Read the model definition and answer for the solid it produces. Units are mm, in the model's axes. Face numbers are marked on the shaded views. A direction names the side the tool comes from. Coordinates: 2 decimals unless noted, no trailing zeros. Write each loop counter-clockwise with the first axis right and the second up, starting at its lowest first coordinate (ties: lowest second). Pieces come first, ordered by that corner, then holes. Notation, with made-up numbers: (21, 57) -> (63, 57) arc R19 cw to (63, 89) -> close; hole circle Ø6 at (-6.75, 76). An arc over 180 degrees is marked (long way). One line per item, written item: value. Start each with the question number.
1. Consider line 1 along Y through (x, z) = (0, 9.5); line 2 along Y through (x, z) = (-2.25, 8). Determine where each line is inside the solid, lowest interval first.
2. For a pull along Y with two mould halves and no side action, classify the marked faces 1, 2 and 3 as pulls with the +Y half, pulls with the -Y half, needs draft (parallel to the pull), parting line crosses it, or undercut.
3. Find section D-D, the plane x = -2. Write down the section's boundary in (y, z).
4. Given P1, Ø5, axis at y = 6, z = 11, coming from the -X side; P2, Ø6.5, axis at x = 0, y = 0, coming from the -Z side; P3, Ø10, axis at y = -9.5, z = 9, coming from the +X side; P4, Ø10, axis at x = -10, y = -1.5, coming from the +Z side, each flat-ended and moving along its own axis, determine where each tip first touches the part or whether it passes through.
5. For the marked faces 4 and 5, determine the directions among +Z, -Z, +X, -X, +Y, -Y from which every point of the face is accessible in a straight line to the end or side of a thin tool.
6. Find section C-C, the plane x = -11. Write down the section's boundary in (y, z).
7. Find section B-B, the plane z = 20.75. Write down the section's boundary in (x, y), and give its area (3 significant figures).
8. Find section A-A, the plane y = 10.5. Write down the section's boundary in (x, z), and give its area (3 significant figures).
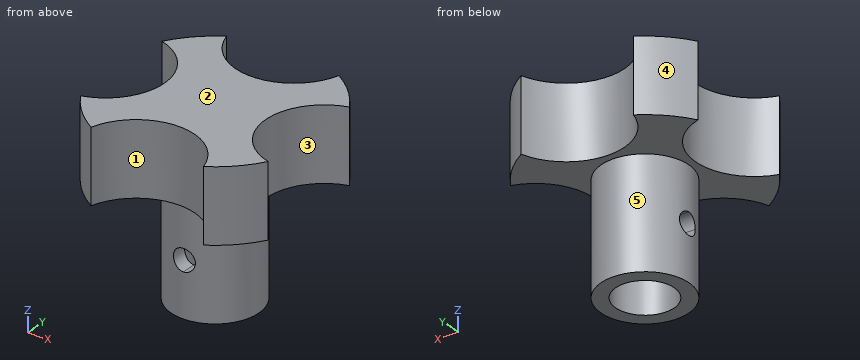
```python
from build123d import *

# Parameters (mm, degrees)
IZIM1_R                     = 6
IZIM1_R_2                   = 4
Y_KSEKLIK_EKSTR_ZYON1_DEPTH = 15
Y_KSEKLIK_EKSTR_ZYON2_DEPTH = 10
KES_EKSTR_ZYON1_DEPTH       = 15
DAIRESEL_KAPLAMA1_COUNT     = 2
DAIRESEL_KAPLAMA1_ANGLE     = 90


with BuildPart() as part:
    # Çizim1 → Yükseklik-Ekstrüzyon1 (new body)
    with BuildSketch(Plane.XY):
        Circle(IZIM1_R)
        Circle(IZIM1_R_2, mode=Mode.SUBTRACT)
    extrude(amount=Y_KSEKLIK_EKSTR_ZYON1_DEPTH)

    # Çizim2 → Yükseklik-Ekstrüzyon2 (add)
    with BuildSketch(Plane.XY.offset(15)):
        with BuildLine():
            ThreePointArc((-7.710310557, 12.866666667), (-10.606601718, 10.606601718), (-12.866666667, 7.710310557))
            ThreePointArc((-12.866666667, 7.710310557), (-7, 0), (-12.866666667, -7.710310557))
            ThreePointArc((-12.866666667, -7.710310557), (-10.606601718, -10.606601718), (-7.710310557, -12.866666667))
            ThreePointArc((-7.710310557, -12.866666667), (0, -7), (7.710310557, -12.866666667))
            ThreePointArc((7.710310557, -12.866666667), (10.606601718, -10.606601718), (12.866666667, -7.710310557))
            ThreePointArc((12.866666667, -7.710310557), (7, 0), (12.866666667, 7.710310557))
            ThreePointArc((12.866666667, 7.710310557), (10.606601718, 10.606601718), (7.710310557, 12.866666667))
            ThreePointArc((7.710310557, 12.866666667), (0, 7), (-7.710310557, 12.866666667))
        make_face()
    extrude(amount=Y_KSEKLIK_EKSTR_ZYON2_DEPTH)

    # Çizim3 → Kes-Ekstrüzyon1 (cut)
    with BuildSketch(Plane(origin=(0, 0, 0), x_dir=(1, 0, 0), z_dir=(0, 1, 0))):
        with BuildLine():
            ThreePointArc((1.5, -7.5), (1.060660172, -6.439339828), (0, -6))
            Line((0, -6), (0, -9))
            ThreePointArc((0, -9), (1.060660172, -8.560660172), (1.5, -7.5))
        make_face()
        with BuildLine():
            Line((0, -9), (0, -6))
            ThreePointArc((0, -6), (-1.5, -7.5), (0, -9))
        make_face()
    kes_ekstr_zyon1 = extrude(amount=-KES_EKSTR_ZYON1_DEPTH, mode=Mode.SUBTRACT)

    # Dairesel Kaplama1: Kes-Ekstrüzyon1 ×2 about axis
    dairesel_kaplama1_axis = Axis((0, 0, 15), (0, 0, -1))
    for i in range(1, DAIRESEL_KAPLAMA1_COUNT):
        add(kes_ekstr_zyon1.rotate(dairesel_kaplama1_axis, i * DAIRESEL_KAPLAMA1_ANGLE / (DAIRESEL_KAPLAMA1_COUNT - 1)), mode=Mode.SUBTRACT)


solid = part.part
```
Answer block:
1. line 1: y = -6 to -4, 4 to 6
1. line 2: y = -5.56 to -3.31, 3.31 to 5.56
2. face 1: pulls with the -Y half
2. face 2: needs draft
2. face 3: undercut
3. outline: (-7.25, 15) -> (-5.66, 15) -> (-5.66, 0) -> (-3.46, 0) -> (-3.46, 15) -> (3.46, 15) -> (3.46, 0) -> (5.66, 0) -> (5.66, 15) -> (7.25, 15) -> (7.25, 25) -> (-7.25, 25) -> close
4. P1: stops at x = -4.87
4. P2: stops at z = 15
4. P3: stops at x = 3.97
4. P4: stops at z = 25
5. face 4: +Z, -Z, -X, +Y
5. face 5: -Z
6. outline: (-10.2, 15) -> (-6.93, 15) -> (-6.93, 25) -> (-10.2, 25) -> close; (6.93, 15) -> (10.2, 15) -> (10.2, 25) -> (6.93, 25) -> close
7. outline: (-12.87, -7.71) arc R15 ccw to (-7.71, -12.87) arc R8 cw to (7.71, -12.87) arc R15 ccw to (12.87, -7.71) arc R8 cw to (12.87, 7.71) arc R15 ccw to (7.71, 12.87) arc R8 cw to (-7.71, 12.87) arc R15 ccw to (-12.87, 7.71) arc R8 cw to start
7. area: 351 mm2
8. outline: (-10.71, 15) -> (-6.61, 15) -> (-6.61, 25) -> (-10.71, 25) -> close; (6.61, 15) -> (10.71, 15) -> (10.71, 25) -> (6.61, 25) -> close
8. area: 82.0 mm2
